```python
from build123d import *

# Parameters (mm, degrees)
BOSS_EXTRUDE1_DEPTH      = 70
BOSS_EXTRUDE1_DEPTH_BACK = 70
SKETCH1_R                = 15
SKETCH2_W                = 100
SKETCH2_H                = 80
CUT_EXTRUDE1_DEPTH       = 159.429795178
SKETCH3_W                = 50
SKETCH3_H                = 35
CUT_EXTRUDE2_DEPTH       = 116.433963806
FILLET1_R                = 10
RIB1_REACH               = 139.931
SKETCH4_WALL_W           = 322.583644032
SKETCH4_WALL_H           = 15


with BuildPart() as part:
    # Sketch1 → Boss-Extrude1 (new, two sides: drawn at the far end of the back side and taken through both)
    with BuildSketch(Plane.XY.offset(-BOSS_EXTRUDE1_DEPTH_BACK)):
        with BuildLine():
            Line((-40, 70), (-45, 70))
            Line((-45, 70), (-45, 0))
            Line((-45, 0), (45, 0))
            Line((45, 0), (45, 70))
            Line((45, 70), (40, 70))
            ThreePointArc((40, 70), (0, 110), (-40, 70))
        make_face()
        with Locations((0, 70)):
            Circle(SKETCH1_R, mode=Mode.SUBTRACT)
    extrude(amount=BOSS_EXTRUDE1_DEPTH + BOSS_EXTRUDE1_DEPTH_BACK)

    # Sketch2 → Cut-Extrude1 (cut, through all)
    with BuildSketch(Plane.ZY.offset(45)):
        with Locations((-20, 70)):
            Rectangle(SKETCH2_W, SKETCH2_H)
    extrude(amount=-CUT_EXTRUDE1_DEPTH, mode=Mode.SUBTRACT)

    # Sketch3 → Cut-Extrude2 (cut, through all)
    with BuildSketch(Plane(origin=(0, 30, 0), x_dir=(1, 0, 0), z_dir=(0, 1, 0))):
        with Locations((0, 52.5)):
            Rectangle(SKETCH3_W, SKETCH3_H)
    extrude(amount=-CUT_EXTRUDE2_DEPTH, mode=Mode.SUBTRACT)

    # Fillet1
    fillet1_edges = [part.edges().sort_by_distance(p)[0] for p in [
        (-25, 15, -35),
        (25, 15, -35),
    ]]
    fillet(fillet1_edges, radius=FILLET1_R)

    # Sketch4 wall → Rib1 (add, up to next)
    with BuildSketch(Plane(origin=(0, 40, 10), x_dir=(0, -0.4472135955, -0.894427191), z_dir=(0, 0.894427191, -0.4472135955)), mode=Mode.PRIVATE) as rib1_sk1:
        Rectangle(SKETCH4_WALL_W, SKETCH4_WALL_H)
    rib1_tool1 = extrude(rib1_sk1.sketch, amount=-RIB1_REACH, mode=Mode.PRIVATE) - part.part
    add(rib1_tool1.solids().sort_by_distance((0, 40, 10))[0])


solid = part.part
```
The listing builds one solid part. Answer for the finished solid, in the listing's coordinates (mm). A direction names the side the tool comes from. Coordinates: 2 decimals unless noted, no trailing zeros. Order: outer loops, then holes, each group sorted by start corner. A loop starts at its lowest first (then second) coordinate and runs counter-clockwise, first axis right, second up. Notation, with made-up numbers: M 68,56.5 L 90,56.5 A13 cw 90,80.5 Z; hole C 29,-18.75 d6. An arc over 180 degrees is marked long. Answer as a JSON object with one key per item and string values. Group by question number.
1. Section B-B on z = -55 is taken. Write down the section's boundary in (x, y).
2. Section A-A on x = 0 is taken. Write down the section's boundary in (y, z).
3. Straight lines are drawn through the part: line 1 (Y direction, x = 0, z = 60); line 2 (Y direction, x = 37.5, z = -61.5); line 3 (Z direction, x = 3, y = 28). For each, find the intervals that lie inside material, in ascending order.
4. A tool of negligible diameter and unlimited length cuts with its end or side. For faces 1 (the flat face through (-7.5, 38, 17)), 2 (the flat face through (-25, 15, -57)), 3 (the flat face through (7.5, 38, 17)), 4 (the flat face through (43, 70, 50)), from which of +Z, -Z, +X, -X, +Y, -Y can it reach the whole face along a straight path? Write none if from no direction.
5. Determine the mould class of faces 5 (the cylindrical face through (-21.99, 14.79, -37.85)), 6 (the flat face through (-42, 70, 50)), 7 (the flat face through (-45, 28, 15)) for opening direction X: released by +X, released by -X, zero draft, split by the parting line, or undercut.
6. Flat-ended cylindrical pins translate along their axes: P1, Ø15, axis at x = 1, y = 10.5, coming from the -Z side; P2, Ø24, axis at x = 7, y = 80.5, coming from the -Z side; P3, Ø18, axis at x = 0, y = 70, coming from the -Z side; P4, Ø8, axis at x = 26.5, z = 33.5, coming from the -Y side. Find the tip coordinate at first contact, or state that the pin passes through.
7. Section D-D on z = 3 is taken. Write down the section's boundary in (x, y), then the cut area to 3 significant figures.
8. Section C-C on y = 13 is taken. Write down the section's boundary in (x, z).
Values follow:
{
 "1": {"outline": "M -45,0 L -25,0 L -25,30 L -45,30 Z; M 25,0 L 45,0 L 45,30 L 25,30 Z"},
 "2": {"outline": "M 0,-35 L 30,-35 L 30,-10 L 50,30 L 55,30 L 55,70 L 0,70 Z; M 85,30 L 110,30 L 110,70 L 85,70 Z"},
 "3": {"line 1": "0 to 55, 85 to 110", "line 2": "0 to 30", "line 3": "-35 to 70"},
 "4": {"face 1": "-Z, -X, +Y", "face 2": "-Z, +Y, -Y", "face 3": "-Z, +X, +Y", "face 4": "+Z, -Z, +X, +Y"},
 "5": {"face 5": "undercut", "face 6": "zero draft", "face 7": "released by -X"},
 "6": {"P1": "z = -35", "P2": "z = 30", "P3": "through", "P4": "y = 0"},
 "7": {"outline": "M -45,0 L 45,0 L 45,30 L 7.5,30 L 7.5,36.5 L -7.5,36.5 L -7.5,30 L -45,30 Z", "area": "2,800 mm2"},
 "8": {"outline": "M -45,-70 L -25,-70 L -25,-45 A10 cw -15,-35 L 15,-35 A10 cw 25,-45 L 25,-70 L 45,-70 L 45,70 L -45,70 Z"}
}
